Geometry: final body of the model. Coordinates: model frame, mm. Face numbers are marked on the shaded views. A direction names the side the tool comes from. Give positions to 0.01 mm unless a question says otherwise; leave off trailing zeros. Loops run counter-clockwise (first coordinate to the right, second up) from the corner with the lowest first, then second, coordinate; pieces in that order, holes last.
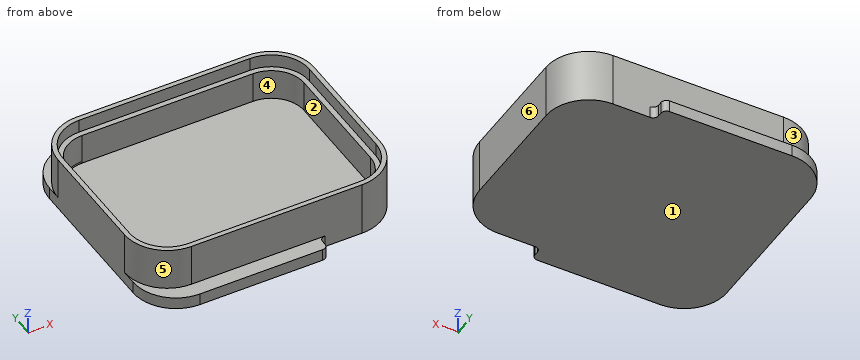
```python
from build123d import *

# Parameters (mm, degrees)
F1_DEPTH     = 10.25
F3_DEPTH     = 2.25
F4_R         = 1
F5_T         = 1.9
F5_T3_DEPTH  = 4.8
F5_T5_DEPTH  = 27.8
F5_T8_ANGLE  = 90.000000001
F5_T10_ANGLE = 90.000000001
F7_DEPTH     = 2.5


# Not quite as in the source:
# - a shell that OpenCascade refuses in one call is made with other operations: the cavity is built on its own and cut out


with BuildPart() as f1:
    # F0 (on Top) → F1 (new body)
    with BuildSketch(Plane.XY):
        with BuildLine():
            Line((16, 19), (-16, 19))
            ThreePointArc((-16, 19), (-21.6568542495, 16.6568542495), (-24, 11))
            Line((-24, 11), (-24, -11))
            ThreePointArc((-24, -11), (-21.6568542495, -16.6568542495), (-16, -19))
            Line((-16, -19), (16, -19))
            ThreePointArc((16, -19), (21.6568542495, -16.6568542495), (24, -11))
            Line((24, -11), (24, 11))
            ThreePointArc((24, 11), (21.6568542495, 16.6568542495), (16, 19))
        make_face()
    extrude(amount=F1_DEPTH)

    # F2 (on Top) → F3 (join)
    with BuildSketch(Plane.XY):
        with BuildLine():
            Line((8, 21.85), (-16, 21.85))
            ThreePointArc((-16, 21.85), (-21.6568542495, 19.5068542495), (-24, 13.85))
            Line((-24, 13.85), (-24, -13.85))
            ThreePointArc((-24, -13.85), (-21.6568542495, -19.5068542495), (-16, -21.85))
            Line((-16, -21.85), (8, -21.85))
            Line((8, -21.85), (8, 21.85))
        make_face()
    extrude(amount=F3_DEPTH)

    # F4
    f4_edges = [f1.edges().sort_by_distance(p)[0] for p in [
        (8, 21.85, 1.125),
        (8, 19, 1.125),
        (8, -19, 1.125),
        (8, -21.85, 1.125),
    ]]
    fillet(f4_edges, radius=F4_R)

    # F5: shell of thickness 1.9, made by hand


with BuildPart() as f5_core1:
    # F5_t2: copy of F1
    add(f1.part)

    # the walls: a layer under each face that stays
    f5_faces = [f5_core1.faces().sort_by_distance(p)[0] for p in [
        (0, 19, 5.125),
        (0, 0, 0),
        (8.2928932188, 19.2928932188, 1.125),
        (21.6568542495, 16.6568542495, 5.125),
        (-18.5, 20.0416666667, 2.25),
        (-21.6568542495, 16.6568542495, 6.25),
        (8, 20.425, 1.125),
        (24, 0, 5.125),
        (21.6568542495, -16.6568542495, 5.125),
        (-4.5, 21.85, 1.125),
        (0, -19, 5.125),
        (-21.6568542495, 19.5068542495, 1.125),
        (8.2928932188, -19.2928932188, 1.125),
        (-24, 0, 5.125),
        (8, -20.425, 1.125),
        (-21.6568542495, -19.5068542495, 1.125),
        (-4.5, -21.85, 1.125),
        (-21.6568542495, -16.6568542495, 6.25),
        (-18.5, -20.0416666667, 2.25),
    ]]
    thicken(f5_faces, amount=-F5_T, mode=Mode.SUBTRACT)

    # F5_s4 → F5_t3 (cut)
    with BuildSketch(Plane.YZ.offset(6.1)):
        Polygon((19.019, 2.269), (17.1, 2.25), (17.1, 0.35), (19, 0.35), align=None)
        Polygon((-19.019, 2.269), (-17.1, 2.25), (-17.1, 0.35), (-19, 0.35), align=None)
    extrude(amount=F5_T3_DEPTH, mode=Mode.SUBTRACT)

    # F5_s6 → F5_t5 (cut)
    with BuildSketch(Plane.YZ.offset(-17.9)):
        Polygon((19.019, 2.269), (17.1, 2.25), (17.1, 0.35), (19, 0.35), align=None)
        Polygon((-19.019, 2.269), (-17.1, 2.25), (-17.1, 0.35), (-19, 0.35), align=None)
    extrude(amount=F5_T5_DEPTH, mode=Mode.SUBTRACT)

    # F5_s7 → F5_t8 (revolve, cut)
    with BuildSketch(Plane.XZ.offset(-11)):
        Polygon((-24.019, 2.269), (-24, 0.35), (-22.1, 0.35), (-22.1, 2.25), align=None)
    revolve(axis=Axis((-16, 11, 2.25), (0, 0, -1)), revolution_arc=F5_T8_ANGLE, mode=Mode.SUBTRACT)

    # F5_s9 → F5_t10 (revolve, cut)
    with BuildSketch(Plane.YZ.offset(-16)):
        Polygon((-19.019, 2.269), (-17.1, 2.25), (-17.1, 0.35), (-19, 0.35), align=None)
    revolve(axis=Axis((-16, -11, 2.25), (0, 0, -1)), revolution_arc=F5_T10_ANGLE, mode=Mode.SUBTRACT)


with BuildPart() as f1_1:
    add(f1.part)

    # what is left inside the walls is the cavity
    f5_cavity = [f5_core1.part.solids().sort_by_distance(p)[0] for p in [
        (0, -5.7, 10.231),
    ]]
    add(f5_cavity, mode=Mode.SUBTRACT)

    # F6 (on face) → F7 (cut)
    with BuildSketch(Plane.XY.offset(10.25)):
        with BuildLine():
            Line((23.1, -11), (23.1, 11))
            ThreePointArc((23.1, 11), (21.0204581464, 16.0204581464), (16, 18.1))
            Line((16, 18.1), (-16, 18.1))
            ThreePointArc((-16, 18.1), (-21.0204581464, 16.0204581464), (-23.1, 11))
            Line((-23.1, 11), (-23.1, -11))
            ThreePointArc((-23.1, -11), (-21.0204581464, -16.0204581464), (-16, -18.1))
            Line((-16, -18.1), (16, -18.1))
            ThreePointArc((16, -18.1), (21.0204581464, -16.0204581464), (23.1, -11))
        make_face()
        with BuildLine():
            Line((-22.1, -11), (-22.1, 11))
            ThreePointArc((-22.1, 11), (-20.3133513652, 15.3133513652), (-16, 17.1))
            Line((-16, 17.1), (16, 17.1))
            ThreePointArc((16, 17.1), (20.3133513652, 15.3133513652), (22.1, 11))
            Line((22.1, 11), (22.1, -11))
            ThreePointArc((22.1, -11), (20.3133513652, -15.3133513652), (16, -17.1))
            Line((16, -17.1), (-16, -17.1))
            ThreePointArc((-16, -17.1), (-20.3133513652, -15.3133513652), (-22.1, -11))
        make_face(mode=Mode.SUBTRACT)
    extrude(amount=-F7_DEPTH, mode=Mode.SUBTRACT)


solid = f1_1.part
```
Q1. Section query D-D, the plane z = 1. Return loops of the section in (x, y).
Q2. Section query A-A, the plane z = 9.25. Return loops of the section in (x, y), and give its area (3 significant figures).
Q3. Material intervals for probe 1 along Y at (x, z) = (-12, 9); probe 2 along Y at (x, z) = (-1, 6.25); probe 3 along X at (y, z) = (-8, 2), sorted ascending.
Q4. Section query B-B, the plane x = -2.5. Return loops of the section in (y, z).
Q5. Reachability of the marked faces 1, 2 and 3 from +Z, -Z, +X, -X, +Y, -Y: full face, straight path, thin tool, end or side. Return the list, or none.
Q6. Pin query (flat end, axial travel): pin 1 Ø4 at (x, y) = (-15.5, 5.5) entering from +Z; pin 2 Ø0.8 at (x, z) = (2, 9) entering from -Y; pin 3 Ø3 at (x, z) = (-4.5, 5.5) entering from +Y. Return the tip coordinate at first contact, or that it passes through.
Q7. Section query C-C, the plane y = -2. Return loops of the section in (x, z).
Q8. Mould query, pull axis Y, two halves, no side actions, for the marked faces 4, 5 and 6. Classes: +Y half, -Y half, draft (parallel to the pull), parting line (faces both ways), or undercut.
Resolved:
1. outline: (-24, -13.85) arc R8 ccw to (-16, -21.85) - (7, -21.85) arc R1 ccw to (8, -20.85) - (8, -20) arc R1 cw to (9, -19) - (16, -19) arc R8 ccw to (24, -11) - (24, 11) arc R8 ccw to (16, 19) - (9, 19) arc R1 cw to (8, 20) - (8, 20.85) arc R1 ccw to (7, 21.85) - (-16, 21.85) arc R8 ccw to (-24, 13.85) - close
2. outline: (-24, -11) arc R8 ccw to (-16, -19) - (16, -19) arc R8 ccw to (24, -11) - (24, 11) arc R8 ccw to (16, 19) - (-16, 19) arc R8 ccw to (-24, 11) - close; hole (-23.1, -11) arc R7.1 ccw to (-16, -18.1) - (16, -18.1) arc R7.1 ccw to (23.1, -11) - (23.1, 11) arc R7.1 ccw to (16, 18.1) - (-16, 18.1) arc R7.1 ccw to (-23.1, 11) - close
2. area: 140 mm2
3. probe 1: y = -19 to -18.1, 18.1 to 19
3. probe 2: y = -19 to -17.1, 17.1 to 19
3. probe 3: x = -24 to -22.1, 22.1 to 24
4. outline: (-21.85, 0) - (21.85, 0) - (21.85, 2.25) - (19, 2.25) - (19, 10.25) - (18.1, 10.25) - (18.1, 7.75) - (17.1, 7.75) - (17.1, 1.9) - (-17.1, 1.9) - (-17.1, 7.75) - (-18.1, 7.75) - (-18.1, 10.25) - (-19, 10.25) - (-19, 2.25) - (-21.85, 2.25) - close
5. face 1: -Z, +X, -X, +Y, -Y
5. face 2: +Z
5. face 3: +Z, -X, +Y
6. pin 1: stops at z = 1.9
6. pin 2: stops at y = -19
6. pin 3: stops at y = 19
7. outline: (-24, 0) - (24, 0) - (24, 10.25) - (23.1, 10.25) - (23.1, 7.75) - (22.1, 7.75) - (22.1, 1.9) - (-22.1, 1.9) - (-22.1, 7.75) - (-23.1, 7.75) - (-23.1, 10.25) - (-24, 10.25) - close
8. face 4: undercut
8. face 5: -Y half
8. face 6: draft
